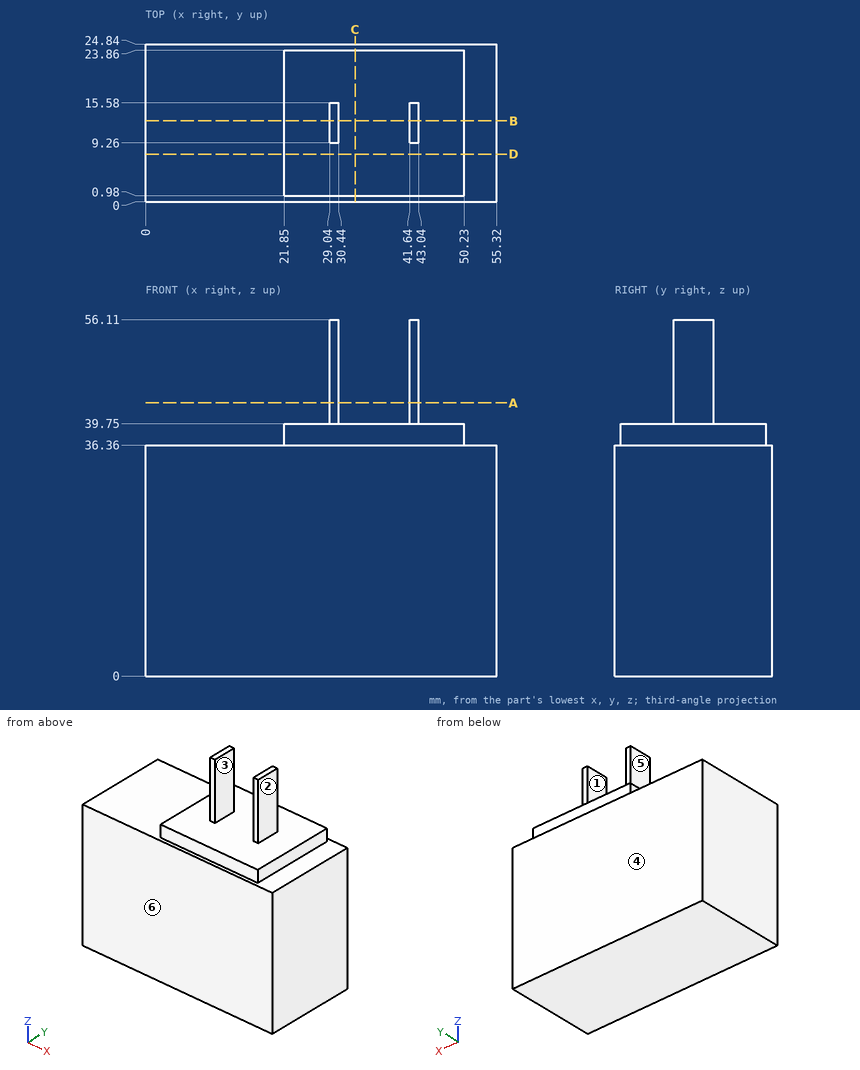
Geometry: see drawing. Coordinates: mm, zero at the bounding-box minimum. A direction names the side the tool comes from. Give positions to 0.01 mm unless a question says otherwise; leave off trailing zeros. Write each loop counter-clockwise with the first axis right and the second up, starting at its lowest first coordinate (ties: lowest second). Pieces come first, ordered by that corner, then holes. Notation, with made-up numbers: M -37.5,-10.5 L -29.5,-10.5 A18 cw -29.5,9.5 Z; hole C 55.5,0.5 d4. An arc over 180 degrees is marked long. Return JSON: item names as keys, results as strings. Group by question number.
1) Draft query along X for the marked faces 1, 2, 3 and 4. Return one class per face: released by +X, released by -X, zero draft, split by the parting line, or undercut.
2) First-contact query: pin 1 Ø3.5 at (x, z) = (37, 38.5) entering from -Y; pin 2 Ø1.9 at (y, z) = (13.5, 45.5) entering from -X; pin 3 Ø2.5 at (y, z) = (17.5, 38) entering from +X. Flat tips, straight axial feed; report the tip coordinate or a pass-through.
3) Ray query, L1, parallel to X at y = 1.75, z = 38.5; L2, parallel to Z at x = 32.5, y = 14.75; L3, parallel to Z at x = 4, y = 3.75. Return the intervals inside material, ascending.
4) Cut plane B-B, the plane y = 12.75. Output: boundary loops of the cut face in (x, z), then the cut area to 3 significant figures.
5) Cut plane A-A, the plane z = 43. Output: boundary loops of the cut face in (x, y).
6) Cut plane D-D, the plane y = 7.5. Output: boundary loops of the cut face in (x, z), then the cut area to 3 significant figures.
7) Cut plane C-C, the plane x = 33. Output: boundary loops of the cut face in (y, z).
8) Set-up query: the marked faces 5 and 6. Return all of +Z, -Z, +X, -X, +Y, -Y with unobstructed straight access to the full face (end or side cutting, diameter ignored); none if empty.
Data:
{
 "1": {"face 1": "undercut", "face 2": "released by +X", "face 3": "undercut", "face 4": "zero draft"},
 "2": {"pin 1": "stops at y = 0.98", "pin 2": "stops at x = 29.04", "pin 3": "stops at x = 50.23"},
 "3": {"L1": "x = 21.85 to 50.23", "L2": "z = 0 to 39.75", "L3": "z = 0 to 36.36"},
 "4": {"outline": "M 0,0 L 55.32,0 L 55.32,36.36 L 50.23,36.36 L 50.23,39.75 L 43.04,39.75 L 43.04,56.11 L 41.64,56.11 L 41.64,39.75 L 30.44,39.75 L 30.44,56.11 L 29.04,56.11 L 29.04,39.75 L 21.85,39.75 L 21.85,36.36 L 0,36.36 Z", "area": "2,150 mm²"},
 "5": {"outline": "M 29.04,9.26 L 30.44,9.26 L 30.44,15.58 L 29.04,15.58 Z; M 41.64,9.26 L 43.04,9.26 L 43.04,15.58 L 41.64,15.58 Z"},
 "6": {"outline": "M 0,0 L 55.32,0 L 55.32,36.36 L 50.23,36.36 L 50.23,39.75 L 21.85,39.75 L 21.85,36.36 L 0,36.36 Z", "area": "2,110 mm²"},
 "7": {"outline": "M 0,0 L 24.84,0 L 24.84,36.36 L 23.86,36.36 L 23.86,39.75 L 0.98,39.75 L 0.98,36.36 L 0,36.36 Z"},
 "8": {"face 5": "+Z, -X, +Y, -Y", "face 6": "+Z, -Z, +X, -X, -Y"}
}
